Input: part model. Units: mm. Frame: model coordinates. Round coordinates to 2 decimals unless told otherwise and drop trailing zeros. Write each loop counter-clockwise with the first axis right and the second up, starting at its lowest first coordinate (ties: lowest second). Pieces come first, ordered by that corner, then holes. Notation, with made-up numbers: M 30,-23.75 L 45,-23.75 A25 cw 45,2.25 Z; hole C 5,34.5 d3. An arc over 180 degrees is marked long. Answer as CSV lines item,"result". Start each with the question number.
```python
from build123d import *

# Parameters (mm, degrees)
SKETCH1_W           = 40
SKETCH1_H           = 9.75
SKETCH1_R           = 1.5
BOSS_EXTRUDE1_DEPTH = 8
CUT_EXTRUDE1_REACH  = 25.645
SKETCH2_R           = 3
SKETCH2_R_2         = 1.5


with BuildPart() as part:
    # Sketch1 → Boss-Extrude1 (new body)
    with BuildSketch(Plane(origin=(0, 0, 0), x_dir=(1, 0, 0), z_dir=(0, 1, 0))):
        Rectangle(SKETCH1_W, SKETCH1_H)
        with Locations(Location((-15.976056303, 0.875, 0), (0, 0, 270))):
            Circle(SKETCH1_R, mode=Mode.SUBTRACT)
        with Locations(Location((15.976056303, 0.875, 0), (0, 0, 90))):
            Circle(SKETCH1_R, mode=Mode.SUBTRACT)
    extrude(amount=BOSS_EXTRUDE1_DEPTH)

    # Sketch2 → Cut-Extrude1 (cut, up to next)
    with BuildSketch(Plane.XY.offset(4.875), mode=Mode.PRIVATE) as cut_extrude1_sk1:
        with Locations((0, 4)):
            Circle(SKETCH2_R)
    cut_extrude1_tool1 = extrude(cut_extrude1_sk1.sketch, amount=-CUT_EXTRUDE1_REACH, mode=Mode.PRIVATE) & part.part
    # Sketch2 → Cut-Extrude1 (cut, up to next)
    with BuildSketch(Plane.XY.offset(4.875), mode=Mode.PRIVATE) as cut_extrude1_sk2:
        with Locations((8.5, 4)):
            Circle(SKETCH2_R_2)
    cut_extrude1_tool2 = extrude(cut_extrude1_sk2.sketch, amount=-CUT_EXTRUDE1_REACH, mode=Mode.PRIVATE) & part.part
    # Sketch2 → Cut-Extrude1 (cut, up to next)
    with BuildSketch(Plane.XY.offset(4.875), mode=Mode.PRIVATE) as cut_extrude1_sk3:
        with Locations((-8.5, 4)):
            Circle(SKETCH2_R_2)
    cut_extrude1_tool3 = extrude(cut_extrude1_sk3.sketch, amount=-CUT_EXTRUDE1_REACH, mode=Mode.PRIVATE) & part.part
    add(cut_extrude1_tool1.solids().sort_by_distance((0, 4, 4.875))[0], mode=Mode.SUBTRACT)
    add(cut_extrude1_tool2.solids().sort_by_distance((8.5, 4, 4.875))[0], mode=Mode.SUBTRACT)
    add(cut_extrude1_tool3.solids().sort_by_distance((-8.5, 4, 4.875))[0], mode=Mode.SUBTRACT)


solid = part.part
```
Item 1: Cut plane C-C, the plane y = 6.5. Return loops of the section in (x, z) (3 decimals).
Item 2: Cut plane D-D, the plane z = 0. Return loops of the section in (x, y).
Item 3: Pin query (flat end, axial travel): pin 1 Ø1.8 at (x, z) = (-15.98, -0.88) entering from -Y. Return the tip coordinate at first contact, or that it passes through.
Item 4: Line query: line 1 (Y direction, x = 0, z = -3); line 2 (X direction, y = 3, z = 2); line 3 (Y direction, x = 8.5, z = 0). Output: solid intervals per line, ascending. Write a range as [from, to].
Item 5: Cut plane A-A, the plane y = 3.25. Return loops of the section in (x, z) (3 decimals), plus the area to 3 significant figures.
Item 6: Cut plane B-B, the plane x = 8.5. Return loops of the section in (y, z) (3 decimals).
Item 7: Draft query along X for faces 1 (the face through (14.49, 3.94, -0.68)), 2 (the face through (0, 8, 0)), 3 (the face through (-20, 4, 0)). Return one class per face: +X half, -X half, draft (parallel to the pull), parting line (faces both ways), or undercut.
Results list:
1,outline,"M -20,-4.875 L -1.658,-4.875 L -1.658,4.875 L -20,4.875 Z; M 1.658,-4.875 L 20,-4.875 L 20,4.875 L 1.658,4.875 Z; hole C -15.976,-0.875 d3; hole C 15.976,-0.875 d3"
2,outline,"M -20,0 L -17.19,0 L -17.19,8 L -20,8 Z; M -14.76,0 L 14.76,0 L 14.76,8 L -14.76,8 Z; M 17.19,0 L 20,0 L 20,8 L 17.19,8 Z; hole C -8.5,4 d3; hole C 0,4 d6; hole C 8.5,4 d3"
3,pin 1,"through"
4,line 1,"[0, 1], [7, 8]"
4,line 2,"[-20, -9.62], [-7.38, -2.83], [2.83, 7.38], [9.62, 20]"
4,line 3,"[0, 2.5], [5.5, 8]"
5,outline,"M -20,-4.875 L -9.799,-4.875 L -9.799,4.875 L -20,4.875 Z; M -7.201,-4.875 L -2.905,-4.875 L -2.905,4.875 L -7.201,4.875 Z; M 2.905,-4.875 L 7.201,-4.875 L 7.201,4.875 L 2.905,4.875 Z; M 9.799,-4.875 L 20,-4.875 L 20,4.875 L 9.799,4.875 Z; hole C -15.976,-0.875 d3; hole C 15.976,-0.875 d3"
5,area,"269 mm²"
6,outline,"M 0,-4.875 L 2.5,-4.875 L 2.5,4.875 L 0,4.875 Z; M 5.5,-4.875 L 8,-4.875 L 8,4.875 L 5.5,4.875 Z"
7,face 1,"undercut"
7,face 2,"draft"
7,face 3,"-X half"
